```python
from build123d import *

# Parameters (mm, degrees)
SKETCH1_R                      = 32.5
BOSS_EXTRUDE1_DEPTH            = 10
SKETCH2_R                      = 32.5
SKETCH2_R_2                    = 31
BOSS_EXTRUDE2_DEPTH            = 3
CUT_EXTRUDE1_DEPTH             = 3
CUT_EXTRUDE1_DEPTH_BACK        = 48.037219306
SKETCH3_W                      = 39.818487818
SKETCH3_H                      = 10
FILLET1_R                      = 5
F_3_8_3_8_DIAMETER_HOLE1_D     = 3.8
F_3_8_3_8_DIAMETER_HOLE1_DEPTH = 10
F_3_8_3_8_DIAMETER_HOLE1_TIP   = 1.141635176
SKETCH6_R                      = 20
CUT_EXTRUDE2_DEPTH             = 10


with BuildPart() as part:
    # Sketch1 → Boss-Extrude1 (new body)
    with BuildSketch(Plane(origin=(0, 0, 0), x_dir=(1, 0, 0), z_dir=(0, 1, 0))):
        with Locations(Location((0, 0, 0), (0, 0, 270))):
            Circle(SKETCH1_R)
    extrude(amount=BOSS_EXTRUDE1_DEPTH)

    # Sketch2 → Boss-Extrude2 (add)
    with BuildSketch(Plane(origin=(0, 10, 0), x_dir=(1, 0, 0), z_dir=(0, 1, 0))):
        with Locations(Location((0, 0, 0), (0, 0, 270))):
            Circle(SKETCH2_R)
        with Locations(Location((0, 0, 0), (0, 0, 270))):
            Circle(SKETCH2_R_2, mode=Mode.SUBTRACT)
    extrude(amount=BOSS_EXTRUDE2_DEPTH)

    # Sketch3 → Cut-Extrude1 (cut, two sides: drawn at the far end of the back side and taken through both)
    with BuildSketch(Plane(origin=(0, 10, 0), x_dir=(1, 0, 0), z_dir=(0, 1, 0)).offset(-CUT_EXTRUDE1_DEPTH_BACK)):
        with Locations((19.909243909, 0)):
            Rectangle(SKETCH3_W, SKETCH3_H)
    extrude(amount=CUT_EXTRUDE1_DEPTH + CUT_EXTRUDE1_DEPTH_BACK, mode=Mode.SUBTRACT)

    # Fillet1
    fillet1_edges = [part.edges().sort_by_distance(p)[0] for p in [
        (0, 5, 5),
        (0, 5, -5),
    ]]
    fillet(fillet1_edges, radius=FILLET1_R - 0.0001)  # a hair under: the kernel refuses the full size

    # Ø3.8 (3.8) Diameter Hole1
    with Locations(Plane(origin=(0, 10, 0), x_dir=(1, 0, 0), z_dir=(0, 1, 0))):
        with Locations((0, 26), (0, -26)):
            Hole(F_3_8_3_8_DIAMETER_HOLE1_D / 2, depth=F_3_8_3_8_DIAMETER_HOLE1_DEPTH)
            with Locations((0, 0, -(F_3_8_3_8_DIAMETER_HOLE1_DEPTH + F_3_8_3_8_DIAMETER_HOLE1_TIP / 2))):  # 118° drill point
                Cone(0, F_3_8_3_8_DIAMETER_HOLE1_D / 2, F_3_8_3_8_DIAMETER_HOLE1_TIP, mode=Mode.SUBTRACT)

    # Sketch6 → Cut-Extrude2 (cut)
    with BuildSketch(Plane(origin=(0, 10, 0), x_dir=(1, 0, 0), z_dir=(0, 1, 0))):
        Circle(SKETCH6_R)
    extrude(amount=-CUT_EXTRUDE2_DEPTH, mode=Mode.SUBTRACT)


solid = part.part
```
Source: CAD feature listing. Evaluate the final solid. Frame: model axes, mm. A direction names the side the tool comes from. Coordinates: 2 decimals unless noted, no trailing zeros. Order: outer loops, then holes, each group sorted by start corner. A loop starts at its lowest first (then second) coordinate and runs counter-clockwise, first axis right, second up. Notation, with made-up numbers: (55, 20.25) - (103, 20.25) arc R14 ccw to (103, 33.25) - close; hole circle Ø5 at (53, 18.5). An arc over 180 degrees is marked (long way). One line per item, written item: value.
1) Contact query for flat-ended pins moving along their axis: pin 1 (4 mm diameter, centred on y = 9, z = -20.5, fed in from -X); pin 2 (6.5 mm diameter, centred on x = 25.5, y = 5.5, fed in from -Z); pin 3 (1 mm diameter, centred on x = -25.5, y = 4.5, fed in from -Z); pin 4 (1 mm diameter, centred on x = -19, z = 13.5, fed in from -Y). Output: stop coordinate, or through.
Computed values:
pin 1: stops at x = -26.72
pin 2: stops at z = -23.69
pin 3: stops at z = -20.77
pin 4: stops at y = 0
2) Cut plane B-B on z = 9.5. Output: boundary loops of the cut face in (x, y).
Computed values:
outline: (-31.08, 0) - (-17.6, 0) - (-17.6, 10) - (-29.51, 10) - (-29.51, 13) - (-31.08, 13) - close; (17.6, 0) - (31.08, 0) - (31.08, 13) - (29.51, 13) - (29.51, 10) - (17.6, 10) - close
3) Reachability of faces 1 (the face through (0.247, 4.93, -27.884)), 2 (the face through (-30.973, 11.479, -1.293)), 3 (the face through (26, 5, 5)) from +Z, -Z, +X, -X, +Y, -Y: full face, straight path, thin tool, end or side. Return the list, or none.
Computed values:
face 1: +Y, -Y
face 2: +Y
face 3: +X, +Y, -Y
4) Cut plane A-A on x = 0. Output: boundary loops of the cut face in (y, z).
Computed values:
outline: (0, -32.5) - (13, -32.5) - (13, -31) - (10, -31) - (10, -27.9) - (0, -27.9) - close; (0, -24.1) - (10, -24.1) - (10, -20) - (0, -20) - close; (0, 20) - (10, 20) - (10, 24.1) - (0, 24.1) - close; (0, 27.9) - (10, 27.9) - (10, 31) - (13, 31) - (13, 32.5) - (0, 32.5) - close
5) Cut plane D-D on y = 8.75. Output: boundary loops of the cut face in (x, z).
Computed values:
outline: (19.36, -5) arc R20 cw (long way) to (19.36, 5) - (32.11, 5) arc R32.5 ccw (long way) to (32.11, -5) - close; hole circle Ø3.8 at (0, -26); hole circle Ø3.8 at (0, 26)
6) Ray query, line 1 (Z direction, x = 0, y = 4.75); line 2 (Y direction, x = -23.5, z = -18.5); line 3 (Z direction, x = 7.5, y = 4.75). Return the intervals inside material, ascending. Write a range as [from, to].
Computed values:
line 1: z = [-32.5, -27.9], [-24.1, -20], [20, 24.1], [27.9, 32.5]
line 2: y = [0, 10]
line 3: z = [-31.62, -18.54], [18.54, 31.62]
7) Mould query, pull axis Z, two halves, no side actions, for faces 4 (the face through (-32.47, 6.41, -1.36)), 5 (the face through (-21, 0, 0)), 6 (the face through (-20.3, 10, -0.4)), 7 (the face through (26, 5, -5)). Classes: released by +Z, released by -Z, zero draft, split by the parting line, or undercut.
Computed values:
face 4: split by the parting line
face 5: zero draft
face 6: undercut
face 7: undercut
8) Cut plane C-C on x = 18.5. Output: boundary loops of the cut face in (y, z).
Computed values:
outline: (0, -26.72) - (13, -26.72) - (13, -24.87) - (10, -24.87) - (10, -7.6) - (0, -7.6) - close; (0, 7.6) - (10, 7.6) - (10, 24.87) - (13, 24.87) - (13, 26.72) - (0, 26.72) - close
